Geometry check sheet. Reference: the model listing, model coordinates, mm. A direction names the side the tool comes from. Coordinates: 2 decimals unless noted, no trailing zeros. Loops run counter-clockwise (first coordinate to the right, second up) from the corner with the lowest first, then second, coordinate; pieces in that order, holes last. Notation, with made-up numbers: (76, -38.5) - (127, -38.5) arc R21 ccw to (127, -14.5) - close; hole circle Ø7 at (-26.75, 48). An arc over 180 degrees is marked (long way). Write each question's results on one line, items separated by ' | '. Start each with the question number.
(1) Mould release check, pull along X, two halves, no side actions. Record for faces 3 (the face through (15, 30, 1)), 4 (the face through (35, 20, 1)), 5 (the face through (-17.358, 29.273, 0.986)): pulls with the +X half, pulls with the -X half, needs draft (parallel to the pull), parting line crosses it, or undercut.
(2) Material ranges on probe 1 along Y at (x, z) = (-17, 1.15); probe 2 along Y at (x, z) = (-15.5, 0.6); probe 3 along Y at (x, z) = (36, 1.1), recorded low to high.
(3) Access from +Z, -Z, +X, -X, +Y, -Y to the whole of each face (thin tool, end or side, straight path). Record for faces 1 (the face through (-12, 40, 1)), 2 (the face through (35, -20, 1)).
(4) Go/stop test with a flat-tipped pin: pin 1 Ø1 at (x, z) = (33, 1.5) entering from +Y. Record where the tip stops, or that it passes through.
(5) Sectioned sample at A-A (y = 32). Enter the section's corners in (x, z), plus the area to 3 significant figures.
(6) Sectioned sample at B-B (z = 1.6). Enter the section's corners in (x, y).
(7) Sectioned sample at C-C (y = 23.5). Enter the section's corners in (x, z), plus the area to 3 significant figures.
(8) Sectioned sample at D-D (x = 23). Enter the section's corners in (y, z), plus the area to 3 significant figures.
Autodesk Inventor part; units mm, degrees
ref_plane "YZ Plane" through (0, 0, 0) normal (1, 0, 0) x (0, 1, 0)
ref_plane "XZ Plane" through (0, 0, 0) normal (0, 1, 0) x (-1, 0, 0)
ref_plane "XY Plane" through (0, 0, 0) normal (0, 0, 1) x (1, 0, 0)
sketch "Sketch13" plane through (0, 0, 0) normal (0, 0, 1) x (1, 0, 0)
  line L0 (-25, -40) -> (-25, 40)
  line L1 (-25, 40) -> (0, 40)
  line L2 (0, 40) -> (30, 20)
  line L3 (30, -20) -> (0, -40)
  line L4 (0, -40) -> (-25, -40)
  line L5 (30, 20) -> (40, 20)
  line L6 (40, 20) -> (40, -20)
  line L7 (40, -20) -> (30, -20)
  line L8 (30, -20) -> (30, 20) construction
  circle A0 centre (-17, 32) radius 2.75
  circle A1 centre (-17, -32) radius 2.75
  line L9 (-25, 0) -> (30, 0) construction
  point P0 (0, 0)
  point P1 (40, 0)
  dimension "d95" = 25
  dimension "d96" = 80
  dimension "d97" = 40
  dimension "d98" = 10
  dimension "d100" = 5.5
  dimension "d101" = 8
  dimension "d102" = 8
  dimension "d103" = 30
extrude "Plate5" add sketch "Sketch13" along normal blind 2
fillet "Fillet4" radius 2 4 edges at (-25, 40, 1) (0, 40, 1) (0, -40, 1) (-25, -40, 1)
equation "\"d104\" = Thickness"
equation "\"BendRadius\" = Thickness"
equation "\"BendReliefWidth\" = Thickness"
equation "\"BendReliefDepth\" = 0.5 * Thickness"
equation "\"CornerReliefSize\" = 4 * Thickness"
equation "\"MinimumRemnant\" = 2 * Thickness"
equation "\"TransitionRadius\" = BendRadius"
equation "\"JacobiRadiusSize\" = BendRadius"
equation "\"GapSize\" = Thickness"
properties part number "NDM 7.46 bracket floor stringer"
Outcome:
1) face 3: pulls with the +X half | face 4: needs draft | face 5: undercut
2) probe 1: y = -40 to -34.75, -29.25 to 29.25, 34.75 to 40 | probe 2: y = -40 to -34.3, -29.7 to 29.7, 34.3 to 40 | probe 3: y = -20 to 20
3) face 1: +Z, -Z, +X, -X, +Y | face 2: +Z, -Z, +X, -Y
4) pin 1: stops at y = 20
5) outline: (-25, 0) - (-19.75, 0) - (-19.75, 2) - (-25, 2) - close; (-14.25, 0) - (12, 0) - (12, 2) - (-14.25, 2) - close | area: 63.0 mm2
6) outline: (-25, -38) arc R2 ccw to (-23, -40) - (-0.61, -40) arc R2 ccw to (0.5, -39.66) - (30, -20) - (40, -20) - (40, 20) - (30, 20) - (0.5, 39.66) arc R2 ccw to (-0.61, 40) - (-23, 40) arc R2 ccw to (-25, 38) - close; hole circle Ø5.5 at (-17, -32); hole circle Ø5.5 at (-17, 32)
7) outline: (-25, 0) - (24.75, 0) - (24.75, 2) - (-25, 2) - close | area: 99.5 mm2
8) outline: (-24.67, 0) - (24.67, 0) - (24.67, 2) - (-24.67, 2) - close | area: 98.7 mm2
